from build123d import *

# Parameters (mm, degrees)
SKETCH1_W           = 72
SKETCH1_H           = 33
SKETCH1_R           = 2.75
BOSS_EXTRUDE1_DEPTH = 2.54
FILLET1_R           = 1.5


with BuildPart() as part:
    # Sketch1 → Boss-Extrude1 (new body)
    with BuildSketch(Plane(origin=(0, 0, 0), x_dir=(1, 0, 0), z_dir=(0, 1, 0))):
        Rectangle(SKETCH1_W, SKETCH1_H)
        with Locations(Location((-28, 4.5, 0), (0, 0, 270))):
            Circle(SKETCH1_R, mode=Mode.SUBTRACT)
        with Locations(Location((0, 4.5, 0), (0, 0, 270))):
            Circle(SKETCH1_R, mode=Mode.SUBTRACT)
        with Locations(Location((28, 4.5, 0), (0, 0, 90))):
            Circle(SKETCH1_R, mode=Mode.SUBTRACT)
    extrude(amount=BOSS_EXTRUDE1_DEPTH)

    # Fillet1
    fillet1_edges = [part.edges().sort_by_distance(p)[0] for p in [
        (-36, 1.27, -16.5),
        (36, 1.27, -16.5),
        (36, 1.27, 16.5),
        (-36, 1.27, 16.5),
    ]]
    fillet(fillet1_edges, radius=FILLET1_R)


solid = part.part
Verification items for the finished model (mm, model axes). Round coordinates to 2 decimals unless told otherwise and drop trailing zeros. Order: outer loops, then holes, each group sorted by start corner. A loop starts at its lowest first (then second) coordinate and runs counter-clockwise, first axis right, second up. Notation, with made-up numbers: (29, 68.25) -> (49, 68.25) arc R22 cw to (49, 88.25) -> close; hole circle Ø7 at (49, 56). An arc over 180 degrees is marked (long way). Put each result on its own line as item: value.
1) Section check C-C (y = 1.55). Record the cut outline in (x, z), then the cut area to 3 significant figures.
Final values:
outline: (-36, -15) arc R1.5 ccw to (-34.5, -16.5) -> (34.5, -16.5) arc R1.5 ccw to (36, -15) -> (36, 15) arc R1.5 ccw to (34.5, 16.5) -> (-34.5, 16.5) arc R1.5 ccw to (-36, 15) -> close; hole circle Ø5.5 at (-28, -4.5); hole circle Ø5.5 at (0, -4.5); hole circle Ø5.5 at (28, -4.5)
area: 2,300 mm^2
2) Section check B-B (x = 28). Record the cut outline in (y, z), then the cut area to 4 significant figures.
Final values:
outline: (0, -16.5) -> (2.54, -16.5) -> (2.54, -7.25) -> (0, -7.25) -> close; (0, -1.75) -> (2.54, -1.75) -> (2.54, 16.5) -> (0, 16.5) -> close
area: 69.85 mm^2
3) Material ranges on line 1 (X direction, y = 0.75, z = -4.5); line 2 (Z direction, x = 28, y = 1.35); line 3 (X direction, y = 1.95, z = -3), recorded low to high.
Final values:
line 1: x = -36 to -30.75, -25.25 to -2.75, 2.75 to 25.25, 30.75 to 36
line 2: z = -16.5 to -7.25, -1.75 to 16.5
line 3: x = -36 to -30.3, -25.7 to -2.3, 2.3 to 25.7, 30.3 to 36
4) Section check A-A (z = -4.5). Record the cut outline in (x, y).
Final values:
outline: (-36, 0) -> (-30.75, 0) -> (-30.75, 2.54) -> (-36, 2.54) -> close; (-25.25, 0) -> (-2.75, 0) -> (-2.75, 2.54) -> (-25.25, 2.54) -> close; (2.75, 0) -> (25.25, 0) -> (25.25, 2.54) -> (2.75, 2.54) -> close; (30.75, 0) -> (36, 0) -> (36, 2.54) -> (30.75, 2.54) -> close
5) Mould release check, pull along X, two halves, no side actions. Record for faces 1 (the flat face through (0, 1, 16.5)), 2 (the cylindrical face through (25.273, 1.252, -4.142)), 3 (the cylindrical face through (-35.57, 1.29, 16.05)): +X half, -X half, draft (parallel to the pull), parting line (faces both ways), or undercut.
Final values:
face 1: draft
face 2: undercut
face 3: -X half
